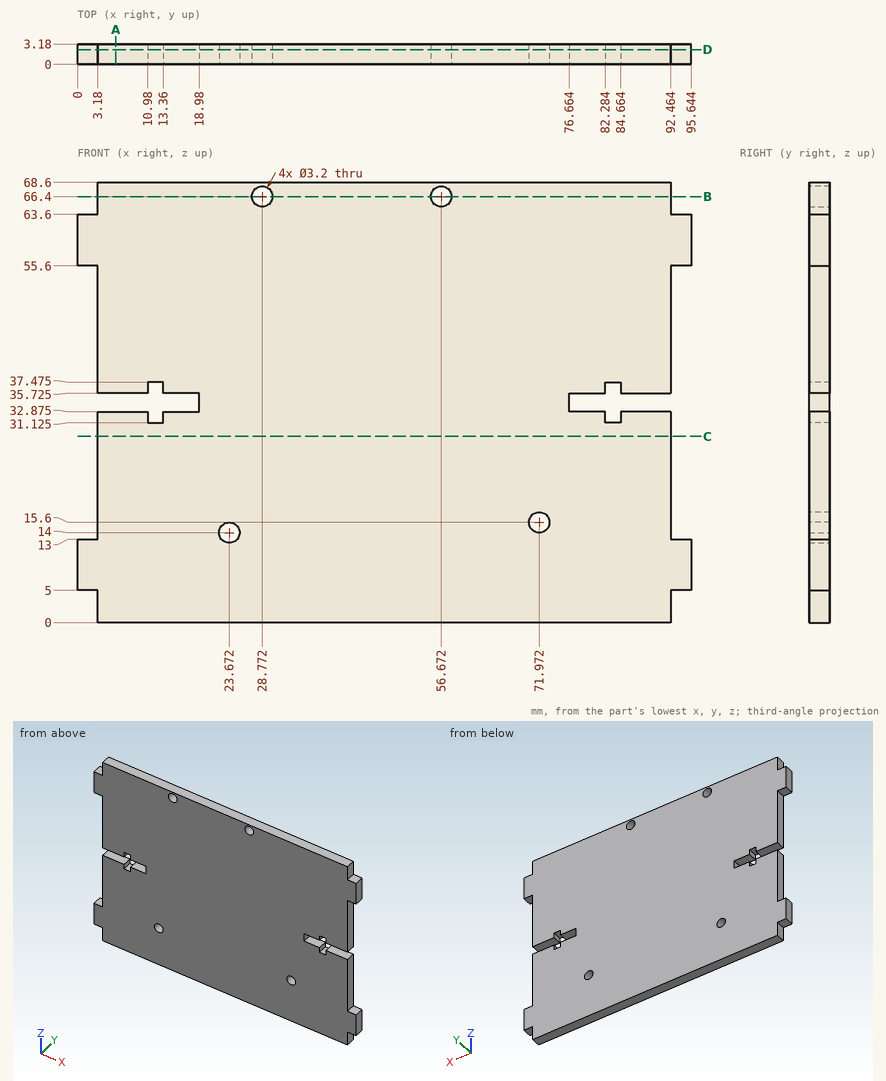
Verification items for this drawing (mm, ordinates from the low corner). Coordinates: 2 decimals unless noted, no trailing zeros. Order: outer loops, then holes, each group sorted by start corner. A loop starts at its lowest first (then second) coordinate and runs counter-clockwise, first axis right, second up. Notation, with made-up numbers: (-14, 47) -> (21, 47) arc R19 cw to (21, 76) -> close; hole circle Ø2 at (44.5, -39.5). An arc over 180 degrees is marked (long way). Put each result on its own line as item: value. Start each with the question number.
1. Go/stop test with flat-tipped pins: pin 1 Ø1.6 at (y, z) = (1, 25) entering from +X; pin 2 Ø1 at (x, y) = (1.5, 1.5) entering from -Z; pin 3 Ø1 at (y, z) = (1, 2) entering from -X. Record where each tip stops, or that it passes through.
2. Material ranges on L1, parallel to X at y = 1.75, z = 66.4; L2, parallel to Z at x = 90, y = 1.7 (3 decimals); L3, parallel to Z at x = 13, y = 2.95 (3 decimals), recorded low to high. Write a range as [from, to].
3. Cross-section at D-D, the plane y = 2.3. Count the separate pieces of the cut face and the enclosed holes in it, then the cut area to 3 significant figures.
4. Cross-section at C-C, the plane z = 29. Record the boundary of the cut face in (x, y), then the cut area to 3 significant figures.
5. Cross-section at B-B, the plane z = 66.4. Record the boundary of the cut face in (x, y).
6. Cross-section at A-A, the plane x = 6. Record the boundary of the cut face in (y, z) (3 decimals).
Computed:
1. pin 1: x = 92.46
1. pin 2: z = 5
1. pin 3: x = 3.18
2. L1: [3.18, 27.17], [30.37, 55.07], [58.27, 92.46]
2. L2: [0, 32.875], [35.725, 68.6]
2. L3: [0, 31.125], [37.475, 68.6]
3. separate pieces: 1
3. enclosed holes: 4
3. area: 6,090 mm2
4. outline: (3.18, 0) -> (92.46, 0) -> (92.46, 3.18) -> (3.18, 3.18) -> close
4. area: 284 mm2
5. outline: (3.18, 0) -> (27.17, 0) -> (27.17, 3.18) -> (3.18, 3.18) -> close; (30.37, 0) -> (55.07, 0) -> (55.07, 3.18) -> (30.37, 3.18) -> close; (58.27, 0) -> (92.46, 0) -> (92.46, 3.18) -> (58.27, 3.18) -> close
6. outline: (0, 0) -> (3.18, 0) -> (3.18, 32.875) -> (0, 32.875) -> close; (0, 35.725) -> (3.18, 35.725) -> (3.18, 68.6) -> (0, 68.6) -> close
